Here's how the part is built. I have some questions about the finished solid (model axes, mm). Face numbers are marked on the shaded views. A direction names the side the tool comes from. Coordinates: 2 decimals unless noted, no trailing zeros. Write each loop counter-clockwise with the first axis right and the second up, starting at its lowest first coordinate (ties: lowest second). Pieces come first, ordered by that corner, then holes.
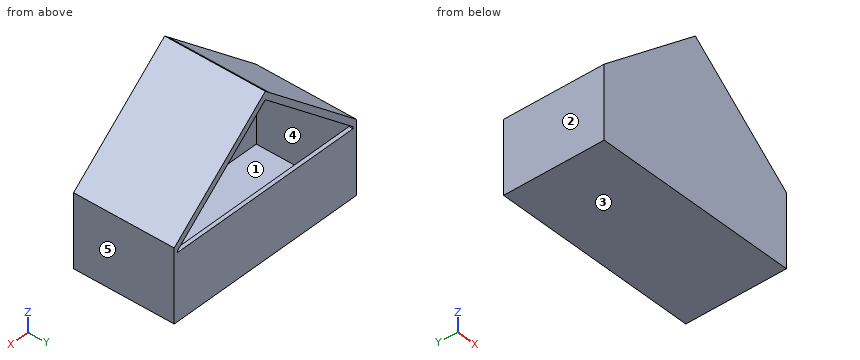
```python
from build123d import *

# Parameters (mm, degrees)
SKETCH1_W           = 1560
SKETCH1_H           = 760
SKETCH1_W_2         = 1500
SKETCH1_H_2         = 700
BOSS_EXTRUDE1_DEPTH = 500
SKETCH2_W           = 1500
SKETCH2_H           = 700
BOSS_EXTRUDE2_DEPTH = 5
SKETCH5_W           = 30
SKETCH5_H           = 760
BOSS_EXTRUDE3_DEPTH = 50
CUT_EXTRUDE1_REACH  = 1260.086
SKETCH7_W           = 46.097722286
SKETCH7_H           = 760
BOSS_EXTRUDE4_DEPTH = 1709
SKETCH8_W           = 30
SKETCH8_H           = 760
BOSS_EXTRUDE5_DEPTH = 50
CUT_EXTRUDE2_REACH  = 2012.771
BOSS_EXTRUDE6_REACH = 2092.258
SKETCH11_W          = 46.097722286
SKETCH11_H          = 760
CUT_EXTRUDE4_DEPTH  = 1023
CUT_EXTRUDE5_DEPTH  = 1023
BOSS_EXTRUDE7_REACH = 1199.247
SKETCH14_W          = 1500
SKETCH14_H          = 30


with BuildPart() as part:
    # Sketch1 → Boss-Extrude1 (new body)
    with BuildSketch(Plane.XY):
        with Locations((58.260712741, 83.006069765)):
            Rectangle(SKETCH1_W, SKETCH1_H)
        with Locations((58.260712741, 83.006069765)):
            Rectangle(SKETCH1_W_2, SKETCH1_H_2, mode=Mode.SUBTRACT)
    extrude(amount=BOSS_EXTRUDE1_DEPTH)

    # Sketch2 → Boss-Extrude2 (add)
    with BuildSketch(Plane.XY):
        with Locations((58.260712741, 83.006069765)):
            Rectangle(SKETCH2_W, SKETCH2_H)
    extrude(amount=BOSS_EXTRUDE2_DEPTH)

    # Sketch5 → Boss-Extrude3 (add)
    with BuildSketch(Plane.XY.offset(500)):
        with Locations((823.260712741, 83.006069765)):
            Rectangle(SKETCH5_W, SKETCH5_H)
    extrude(amount=BOSS_EXTRUDE3_DEPTH)

    # Sketch6 → Cut-Extrude1 (cut, up to next)
    with BuildSketch(Plane(origin=(0, 463.006069765, 0), x_dir=(1, 0, 0), z_dir=(0, 1, 0)), mode=Mode.PRIVATE) as cut_extrude1_sk1:
        Polygon((838.260712741, -550), (808.260712741, -515), (808.260712741, -550), align=None)
    cut_extrude1_tool1 = extrude(cut_extrude1_sk1.sketch, amount=-CUT_EXTRUDE1_REACH, mode=Mode.PRIVATE) & part.part
    add(cut_extrude1_tool1.solids().sort_by_distance((818.260713, 463.00607, 538.333333))[0], mode=Mode.SUBTRACT)

    # Sketch7 → Boss-Extrude4 (add)
    with BuildSketch(Plane(origin=(211.467940286, 0, -181.258234531), x_dir=(0.6507913734559673, 0, 0.7592566023652978), z_dir=(-0.7592566023652978, 0, 0.6507913734559673))):
        with Locations((940.075110717, 83.006069765)):
            Rectangle(SKETCH7_W, SKETCH7_H)
    extrude(amount=BOSS_EXTRUDE4_DEPTH)

    # Sketch8 → Boss-Extrude5 (add)
    with BuildSketch(Plane.XY.offset(500)):
        with Locations((-706.739287259, 83.006069765)):
            Rectangle(SKETCH8_W, SKETCH8_H)
    extrude(amount=BOSS_EXTRUDE5_DEPTH)

    # Sketch10 → Cut-Extrude2 (cut, up to next)
    with BuildSketch(Plane(origin=(0, 463.006069765, 0), x_dir=(1, 0, 0), z_dir=(0, 1, 0)), mode=Mode.PRIVATE) as cut_extrude2_sk1:
        Polygon((-691.739287259, -550), (-691.739287259, -515), (-721.739287259, -550), align=None)
    cut_extrude2_tool1 = extrude(cut_extrude2_sk1.sketch, amount=-CUT_EXTRUDE2_REACH, mode=Mode.PRIVATE) & part.part
    add(cut_extrude2_tool1.solids().sort_by_distance((-701.739287, 463.00607, 538.333333))[0], mode=Mode.SUBTRACT)

    # Boss-Extrude6: up to this plane
    boss_extrude6_end = Plane(origin=(-489.308820701, 463.006069765, 1627.202457236), z_dir=(0.6507913734559673, 0, 0.7592566023652978))
    # Sketch11 → Boss-Extrude6 (add, up to the surface)
    with BuildSketch(Plane(origin=(-144.296765596, 0, -123.682941939), x_dir=(0.6507913734559686, 0, -0.7592566023652966), z_dir=(0.7592566023652966, 0, 0.6507913734559686)), mode=Mode.PRIVATE) as boss_extrude6_sk1:
        with Locations((-864.24397219, 83.006069765)):
            Rectangle(SKETCH11_W, SKETCH11_H)
    boss_extrude6_tool1 = split(extrude(boss_extrude6_sk1.sketch, amount=BOSS_EXTRUDE6_REACH, mode=Mode.PRIVATE), bisect_by=boss_extrude6_end, keep=Keep.BOTH, mode=Mode.PRIVATE)
    add(boss_extrude6_tool1.solids().sort_by_distance((-706.739287, 83.00607, 532.5))[0])

    # Sketch12 → Cut-Extrude4 (cut)
    with BuildSketch(Plane(origin=(0, 463.006069765, 0), x_dir=(1, 0, 0), z_dir=(0, 1, 0))):
        Polygon((55.536353767, -1220.906593407), (-459.308820701, -1662.202457236), (-489.308820701, -1627.202457236), (22.844046075, -1188.214285714), align=None)
    extrude(amount=-CUT_EXTRUDE4_DEPTH, mode=Mode.SUBTRACT)

    # Sketch13 → Cut-Extrude5 (cut)
    with BuildSketch(Plane(origin=(0, 463.006069765, 0), x_dir=(1, 0, 0), z_dir=(0, 1, 0))):
        Polygon((22.844046075, -1188.214285714), (58.260712741, -1218.571428571), (55.536353767, -1220.906593407), align=None)
    extrude(amount=-CUT_EXTRUDE5_DEPTH, mode=Mode.SUBTRACT)

    # Sketch14 → Boss-Extrude7 (add, up to next)
    with BuildSketch(Plane.XY.offset(500), mode=Mode.PRIVATE) as boss_extrude7_sk1:
        with Locations((58.260712741, -281.993930235)):
            Rectangle(SKETCH14_W, SKETCH14_H)
    boss_extrude7_tool1 = extrude(boss_extrude7_sk1.sketch, amount=BOSS_EXTRUDE7_REACH, mode=Mode.PRIVATE) - part.part
    add(boss_extrude7_tool1.solids().sort_by_distance((58.260713, -281.99393, 500))[0])


solid = part.part
```
1) Will these pins go through, and if not, where does the flat tip stop? pin 1 (1 mm diameter, centred on x = -321, y = -73.5, fed in from +Z); pin 2 (9 mm diameter, centred on x = -292, y = 454.5, fed in from +Z); pin 3 (3 mm diameter, centred on y = 323, z = 954.5, fed in from +X).
Values follow:
pin 1: stops at z = 893.92
pin 2: stops at z = 922.21
pin 3: stops at x = 368.09
2) We'd pull the mould along Z, two halves only. Please class the marked faces 1, 2 and 3: pulls with the +Z half, pulls with the -Z half, needs draft (parallel to the pull), parting line crosses it, or undercut.
Values follow:
face 1: undercut
face 2: needs draft
face 3: pulls with the -Z half
3) Imagine slicing it at D-D on z = 880. Please give me the cut outline in (x, y), then the cut area to 3 significant figures.
Values follow:
outline: (-336.74, -296.99) - (453.26, -296.99) - (453.26, 463.01) - (382.43, 463.01) - (382.43, -266.99) - (-265.91, -266.99) - (-265.91, 463.01) - (-336.74, 463.01) - close
area: 127,000 mm2
4) I need wall thicknesses on probe 1 along Y at (x, z) = (571, 54); probe 2 along X at (y, z) = (-163, 329.5); probe 3 along X at (y, z) = (102, 825.5). Which ranges of each line are inside material? Lowest first, please.
Values follow:
probe 1: y = -296.99 to -266.99, 433.01 to 463.01
probe 2: x = -721.74 to -691.74, 808.26 to 838.26
probe 3: x = -400.32 to -329.49, 446.01 to 516.84
5) Imagine slicing it at B-B on y = 312. Please give me the cut outline in (x, z).
Values follow:
outline: (-721.74, 0) - (838.26, 0) - (838.26, 550) - (58.26, 1218.57) - (-721.74, 550) - close; hole (-691.74, 5) - (808.26, 5) - (808.26, 515) - (58.26, 1157.86) - (-691.74, 515) - close
6) Imagine slicing it at C-C on x = 357. Please give me the cut outline in (y, z).
Values follow:
outline: (-296.99, 0) - (463.01, 0) - (463.01, 500) - (433.01, 500) - (433.01, 5) - (-266.99, 5) - (-266.99, 901.79) - (463.01, 901.79) - (463.01, 962.51) - (-296.99, 962.51) - close
7) Imagine slicing it at A-A on z = 468.5. Please give me the cut outline in (x, y), then the cut area to 3 significant figures.
Values follow:
outline: (-721.74, -296.99) - (838.26, -296.99) - (838.26, 463.01) - (-721.74, 463.01) - close; hole (-691.74, -266.99) - (808.26, -266.99) - (808.26, 433.01) - (-691.74, 433.01) - close
area: 136,000 mm2
8) On a 3-axis mill with a long thin cutter (end or side, diameter ignored), from which of +Z, -Z, +X, -X, +Y, -Y can I reach the whole of each face in a straight line? I mean the marked faces 4 and 5. Say none if no direction works.
Values follow:
face 4: none
face 5: +Z, -Z, +X, +Y, -Y
